```python
from build123d import *

# Parameters (mm, degrees)
F0_W     = 127
F0_H     = 127
F1_DEPTH = 190.5
F2_DEPTH = 127
F4_DEPTH = 127
F8_DEPTH = 76.2


with BuildPart() as f1:
    # F0 (on Top) → F1 (new body)
    with BuildSketch(Plane.XY):
        with Locations((63.5, 63.5)):
            Rectangle(F0_W, F0_H)
        with Locations((63.5, 190.5)):
            Rectangle(F0_W, F0_H)
    extrude(amount=F1_DEPTH)

    # F0 (on Top) → F2 (join)
    with BuildSketch(Plane.XY):
        Polygon((127, 127), (127, 0), (254, 127), (254, 254), (127, 254), align=None)
        Polygon((254, 127), (127, 0), (254, 0), align=None)
    extrude(amount=F2_DEPTH)

    # F3 (on face) → F4 (cut)
    with BuildSketch(Plane.YZ.offset(127)):
        Polygon((254, 190.5), (127, 190.5), (254, 127), align=None)
    extrude(amount=-F4_DEPTH, mode=Mode.SUBTRACT)

    # F7 (on 3pt) → F8 (cut)
    with BuildSketch(Plane(origin=(84.6666666667, -84.6666666667, 84.6666666667), x_dir=(0.8164965809, 0.4082482905, -0.4082482905), z_dir=(0.5773502692, -0.5773502692, 0.5773502692))):
        Polygon((207.3901315556, 0), (207.3901315556, 179.6051224214), (51.8475328889, 89.8025612107), align=None)
    extrude(amount=F8_DEPTH, mode=Mode.SUBTRACT)


solid = f1.part
```
Can you work these out from the model? Positions are in its coordinate system, mm. A direction names the side the tool comes from. Give positions to 0.01 mm unless a question says otherwise; leave off trailing zeros. Loops run counter-clockwise (first coordinate to the right, second up) from the corner with the lowest first, then second, coordinate; pieces in that order, holes last. Notation, with made-up numbers: M -31,-10.5 L 2,-10.5 A20 ccw 2,7.5 Z; hole C 25,57.5 d8. An arc over 180 degrees is marked long. One line per question, with ' | ' between items. Start each with the question number.
Q1. If we section it at A-A (x = 160.5): Please give me the cut outline in (y, z), plus the area to 3 significant figures.
Q2. If we section it at B-B (y = 147): Please give me the cut outline in (x, z), plus the area to 3 significant figures.
Q3. For pin 1 Ø1.5 at (y, z) = (57, 127.5) entering from +X; pin 2 Ø12 at (y, z) = (42, 157.5) entering from +X, each with a flat end and sliding along its axis, tell me the tip position at first contact or that it passes through.
Q4. For faces 1 (the flat face through (190, 157, 127)), 2 (the flat face through (125, 129, 0)), which set-ups out of +Z, -Z, +X, -X, +Y, -Y let a thin tool reach every point of the face, with its end or its side?
Q5. If we section it at C-C (z = 77.5): Please give me the cut outline in (x, y), plus the area to 3 significant figures.
Q6. If we section it at D-D (z = 159): Please give me the cut outline in (x, y), plus the area to 3 significant figures.
Q7. If I drill on line 1 (Z direction, x = 239.5, y = 194); line 2 (Z direction, x = 71, y = 170.5), over which ranges is the centre line in solid material (lowest first)? Write a range as from..to.
Computed:
1) outline: M 0,0 L 254,0 L 254,127 L 33.5,127 L 0,93.5 Z | area: 31,700 mm²
2) outline: M 0,0 L 254,0 L 254,127 L 127,127 L 127,180.5 L 0,180.5 Z | area: 39,100 mm²
3) pin 1: stops at x = 184.56 | pin 2: stops at x = 127
4) face 1: +Z, +X, +Y, -Y | face 2: -Z, +X, -X, +Y, -Y
5) outline: M 0,0 L 176.5,0 L 254,77.5 L 254,254 L 0,254 Z | area: 61,500 mm²
6) outline: M 0,0 L 127,0 L 127,190 L 0,190 Z | area: 24,100 mm²
7) line 1: z = 0..127 | line 2: z = 0..168.75
